Work out the finished part from the listing and answer in its coordinate system (mm). A direction names the side the tool comes from. Coordinates: 2 decimals unless noted, no trailing zeros. Loops run counter-clockwise (first coordinate to the right, second up) from the corner with the lowest first, then second, coordinate; pieces in that order, holes last. Notation, with made-up numbers: (71.5, -26.75) -> (115.5, -26.75) arc R27 ccw to (115.5, 3.25) -> close; hole circle Ø8 at (-2.5, 65.25). An arc over 180 degrees is marked (long way). One line per question, with ' | ' between items.
```python
from build123d import *

# Parameters (mm, degrees)
SKETCH_1_R               = 8
EXTRUDE_1_DEPTH          = 51
SKETCH_2_R               = 7
CUT_EXTRUDE_1_DEPTH      = 38
CUT_EXTRUDE_2_DEPTH      = 53.239831546
CUT_EXTRUDE_2_DEPTH_BACK = 53.239831546
SKETCH_3_W               = 2.2
SKETCH_3_H               = 22
FILLET_1_R               = 0.5
FILLET_2_R               = 1
SKETCH_5_R               = 1.5
CUT_EXTRUDE_8_DEPTH      = 38
SKETCH_4_R               = 3
EXTRUDE_2_DEPTH          = 58


with BuildPart() as part:
    # 草图1 → 凸台-拉伸1 (new body)
    with BuildSketch(Plane(origin=(0, 0, 0), x_dir=(1, 0, 0), z_dir=(0, 1, 0))):
        with Locations(Location((0, 0, 0), (0, 0, 270))):
            Circle(SKETCH_1_R)
    extrude(amount=EXTRUDE_1_DEPTH)

    # 草图2 → 切除-拉伸1 (cut)
    with BuildSketch(Plane(origin=(0, 51, 0), x_dir=(1, 0, 0), z_dir=(0, 1, 0))):
        with Locations(Location((0, 0, 0), (0, 0, 270))):
            Circle(SKETCH_2_R)
    extrude(amount=-CUT_EXTRUDE_1_DEPTH, mode=Mode.SUBTRACT)

    # 草图3 → 切除-拉伸2 (cut, two sides: drawn at the far end of the back side and taken through both)
    with BuildSketch(Plane(origin=(0, 0, 0), x_dir=(0, 0, -1), z_dir=(1, 0, 0)).offset(-CUT_EXTRUDE_2_DEPTH_BACK)):
        with Locations((0, 51)):
            Rectangle(SKETCH_3_W, SKETCH_3_H)
    extrude(amount=CUT_EXTRUDE_2_DEPTH + CUT_EXTRUDE_2_DEPTH_BACK, mode=Mode.SUBTRACT)

    # 圆角1
    fillet_1_edges = [part.edges().sort_by_distance(p)[0] for p in [
        (7.418522654, 51, -1.1),
        (-7.418522654, 51, -1.1),
        (-7.418522654, 51, 1.1),
        (7.418522654, 51, 1.1),
    ]]
    fillet(fillet_1_edges, radius=FILLET_1_R)

    # 圆角2
    fillet_2_edges = [part.edges().sort_by_distance(p)[0] for p in [
        (7.418522654, 40, -1.1),
        (-7.418522654, 40, -1.1),
        (7.418522654, 40, 1.1),
        (-7.418522654, 40, 1.1),
    ]]
    fillet(fillet_2_edges, radius=FILLET_2_R)

    # 草图5 → 切除-拉伸8 (cut)
    with BuildSketch(Plane.XZ):
        with Locations(Location((0, 5.5, 0), (0, 0, 270))):
            Circle(SKETCH_5_R)
    extrude(amount=-CUT_EXTRUDE_8_DEPTH, mode=Mode.SUBTRACT)

    # 草图4 → 凸台-拉伸2 (add)
    with BuildSketch(Plane(origin=(0, 0, 0), x_dir=(-1, 0, 0), z_dir=(0, -1, 0))):
        with Locations(Location((0, 0, 0), (0, 0, 90))):
            Circle(SKETCH_4_R)
    extrude(amount=-EXTRUDE_2_DEPTH)


solid = part.part
```
1) For faces 1 (the face through (7.4, 45.7, 1.1)), 2 (the face through (0.1, 13, -3.2)), 3 (the face through (-7.4, 45.7, 1.1)), determine the directions among +Z, -Z, +X, -X, +Y, -Y from which every point of the face is accessible in a straight line to the end or side of a thin tool.
Check values:
face 1: +X, +Y | face 2: +Y | face 3: -X, +Y
2) Find section C-C (x = 3.75). Write down the section's boundary in (y, z), plus the area to 3 significant figures.
Check values:
outline: (0, -7.07) -> (51, -7.07) -> (51, -5.91) -> (13, -5.91) -> (13, 5.91) -> (51, 5.91) -> (51, 7.07) -> (0, 7.07) -> close | area: 272 mm^2
3) Find the intervals of material crossed by line 1 along X through (y, z) = (22, 0); line 2 along Z through (x, y) = (1.25, 50); line 3 along Z through (x, y) = (0, 6.25), in increasing order.
Check values:
line 1: x = -8 to -7, -3 to 3, 7 to 8 | line 2: z = -7.9 to -6.89, -2.73 to 2.73, 6.89 to 7.9 | line 3: z = -8 to 4, 7 to 8
4) The mould has two halves that part along X. Classify faces 4 (the face through (0.9, 35.18, -2.86)), 5 (the face through (-7.81, 25.14, -1.73)), 6 (the face through (7.4, 45.7, -1.1)): released by +X, released by -X, zero draft, split by the parting line, or undercut.
Check values:
face 4: undercut | face 5: split by the parting line | face 6: zero draft
5) Find section B-B (z = 5.5). Write down the section's boundary in (x, y), plus the area to 3 significant figures.
Check values:
outline: (-5.81, 0) -> (-1.5, 0) -> (-1.5, 13) -> (-4.33, 13) -> (-4.33, 51) -> (-5.81, 51) -> close; (1.5, 0) -> (5.81, 0) -> (5.81, 51) -> (4.33, 51) -> (4.33, 13) -> (1.5, 13) -> close | area: 224 mm^2
6) Flat-ended cylindrical pins translate along their axes: pin 1 (8 mm diameter, centred on x = 3, z = -3, fed in from -Y); pin 2 (0.5 mm diameter, centred on x = 7.5, y = 47, fed in from -Z); pin 3 (0.5 mm diameter, centred on x = 7, y = 45, fed in from +Z); pin 4 (1 mm diameter, centred on y = 45.5, z = 5.5, fed in from -X) (3 decimals). Find the tip coordinate at first contact, or state that the pin passes through.
Check values:
pin 1: stops at y = 0 | pin 2: stops at z = -3.38 | pin 3: stops at z = 4.29 | pin 4: stops at x = -6.245
7) Find section A-A (y = 29.5). Write down the section's boundary in (x, z), plus the area to 3 significant figures.
Check values:
outline: circle Ø16 at (0, 0); circle Ø6 at (0, 0); hole circle Ø14 at (0, 0) | area: 75.4 mm^2
8) Find section D-D (x = 0.75). Write down the section's boundary in (y, z), plus the area to 3 significant figures.
Check values:
outline: (0, -7.96) -> (51, -7.96) -> (51, -6.96) -> (13, -6.96) -> (13, -2.9) -> (58, -2.9) -> (58, 2.9) -> (13, 2.9) -> (13, 4.2) -> (0, 4.2) -> close; (0, 6.8) -> (13, 6.8) -> (13, 6.96) -> (51, 6.96) -> (51, 7.96) -> (0, 7.96) -> close | area: 511 mm^2
